For this review, use the dimensioned drawing (mm, ordinates from the lowest corner) and the shaded views. Coordinates: 2 decimals unless noted, no trailing zeros. Write each loop counter-clockwise with the first axis right and the second up, starting at its lowest first coordinate (ties: lowest second). Pieces come first, ordered by that corner, then holes.
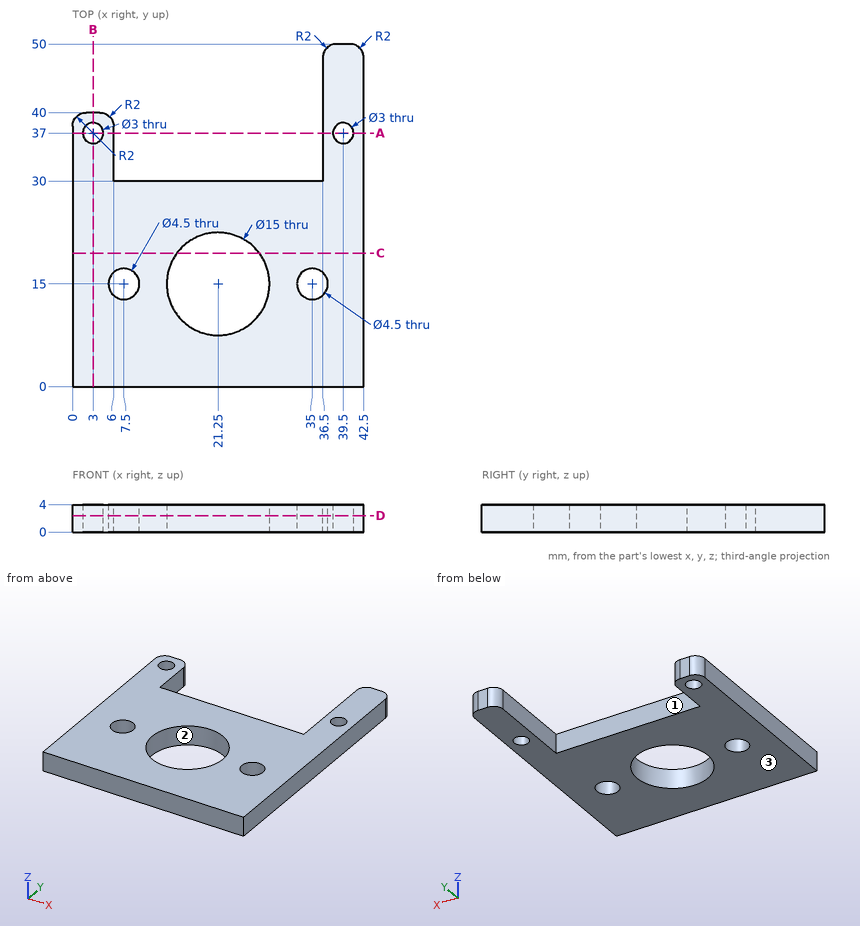
Item 1: Take a section at D-D, the plane z = 2.4. Write out the cut boundary in (x, y), plus the area to 3 significant figures.
Solved:
outline: (0, 0) - (42.5, 0) - (42.5, 48) arc R2 ccw to (40.5, 50) - (38.5, 50) arc R2 ccw to (36.5, 48) - (36.5, 30) - (6, 30) - (6, 38) arc R2 ccw to (4, 40) - (2, 40) arc R2 ccw to (0, 38) - close; hole circle Ø3 at (3, 37); hole circle Ø4.5 at (7.5, 15); hole circle Ø15 at (21.25, 15); hole circle Ø4.5 at (35, 15); hole circle Ø3 at (39.5, 37)
area: 1,230 mm2
Item 2: Take a section at A-A, the plane y = 37. Write out the cut boundary in (x, z).
Solved:
outline: (0, 0) - (1.5, 0) - (1.5, 4) - (0, 4) - close; (4.5, 0) - (6, 0) - (6, 4) - (4.5, 4) - close; (36.5, 0) - (38, 0) - (38, 4) - (36.5, 4) - close; (41, 0) - (42.5, 0) - (42.5, 4) - (41, 4) - close
Item 3: Mouldability with a two-part tool opening along Y and no side actions: class the marked faces 1, 2 and 3 as pulls with the +Y half, pulls with the -Y half, needs draft (parallel to the pull), parting line crosses it, or undercut.
Solved:
face 1: pulls with the +Y half
face 2: undercut
face 3: needs draft
Item 4: Take a section at B-B, the plane x = 3. Write out the cut boundary in (y, z).
Solved:
outline: (0, 0) - (35.5, 0) - (35.5, 4) - (0, 4) - close; (38.5, 0) - (40, 0) - (40, 4) - (38.5, 4) - close
Item 5: To check wall thickness, follow line 1 along X through (y, z) = (35, 2.25); line 2 along Y through (x, z) = (21.25, 2.35); line 3 along X through (y, z) = (16, 0.25). State the ranges of each line that lie inside material, in increasing order.
Solved:
line 1: x = 0 to 6, 36.5 to 42.5
line 2: y = 0 to 7.5, 22.5 to 30
line 3: x = 0 to 5.48, 9.52 to 13.82, 28.68 to 32.98, 37.02 to 42.5
Item 6: For pin 1 (5 mm diameter, centred on x = 3, y = 37, fed in from -Z); pin 2 (1 mm diameter, centred on x = 3, z = 2, fed in from +Y); pin 3 (3.5 mm diameter, centred on x = 7.5, y = 15, fed in from -Z); pin 4 (1 mm diameter, centred on x = 14.5, z = 3.5, fed in from +Y), all flat-tipped, find the tip position at first contact; note any pin that passes through.
Solved:
pin 1: stops at z = 0
pin 2: stops at y = 40
pin 3: passes through
pin 4: stops at y = 30
Item 7: Take a section at C-C, the plane y = 19.5. Write out the cut boundary in (x, z), plus the area to 3 significant figures.
Solved:
outline: (0, 0) - (15.25, 0) - (15.25, 4) - (0, 4) - close; (27.25, 0) - (42.5, 0) - (42.5, 4) - (27.25, 4) - close
area: 122 mm2
